Check sheet for the modelled part. Datum: model origin and axes. Units: mm. Face numbers are marked on the shaded views. A direction names the side the tool comes from. Give positions to 0.01 mm unless a question says otherwise; leave off trailing zeros. Order: outer loops, then holes, each group sorted by start corner. A loop starts at its lowest first (then second) coordinate and runs counter-clockwise, first axis right, second up. Notation, with made-up numbers: (-38, 9) -> (-7, 9) arc R12 ccw to (-7, 24) -> close; hole circle Ø11 at (59.5, -28). An arc over 180 degrees is marked (long way). Write each question's results on one line, items separated by ' | '.
from build123d import *

# Parameters (mm, degrees)
SKETCH1_R           = 16
SKETCH1_R_2         = 7.5
BOSS_EXTRUDE1_DEPTH = 4
SKETCH2_R           = 14
SKETCH2_R_2         = 9.5
CUT_EXTRUDE1_DEPTH  = 0.5
FILLET1_R           = 0.3


with BuildPart() as part:
    # Sketch1 → Boss-Extrude1 (new, symmetric)
    with BuildSketch(Plane.XY):
        Circle(SKETCH1_R)
        Circle(SKETCH1_R_2, mode=Mode.SUBTRACT)
    extrude(amount=BOSS_EXTRUDE1_DEPTH, both=True)

    # Sketch2 → Cut-Extrude1 (cut)
    with BuildSketch(Plane.XY.offset(4)):
        Circle(SKETCH2_R)
        Circle(SKETCH2_R_2, mode=Mode.SUBTRACT)
    cut_extrude1 = extrude(amount=-CUT_EXTRUDE1_DEPTH, mode=Mode.SUBTRACT)

    # Fillet1
    fillet1_edges = [part.edges().sort_by_distance(p)[0] for p in [
        (-16, 0, -4),
        (-16, 0, 4),
        (-7.5, 0, -4),
        (-7.5, 0, 4),
    ]]
    fillet(fillet1_edges, radius=FILLET1_R)

    # Mirror4: Cut-Extrude1 across plane
    add(cut_extrude1.mirror(Plane.XY), mode=Mode.SUBTRACT)


solid = part.part
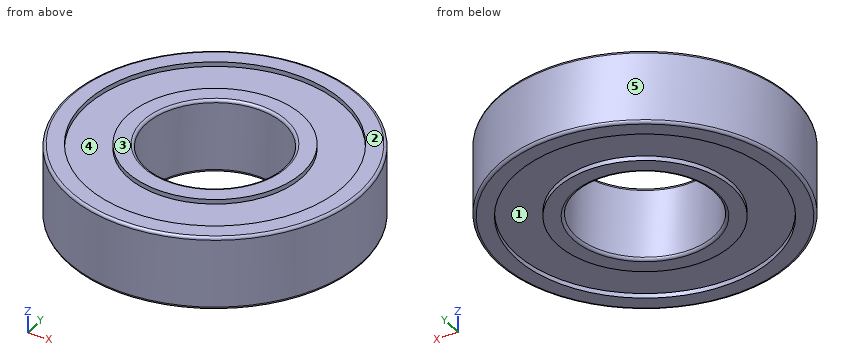
1. Access from +Z, -Z, +X, -X, +Y, -Y to the whole of each face (thin tool, end or side, straight path). Record for the marked faces 1 and 2.
Verdict:
face 1: -Z | face 2: +Z, +X, -X, +Y, -Y
2. Material ranges on probe 1 along Y at (x, z) = (0, -3.6); probe 2 along Z at (x, y) = (8.5, -7); probe 3 along X at (y, z) = (-0.5, 3.75), recorded low to high. Write a range as from..to.
Verdict:
probe 1: y = -16..-14, -9.5..-7.5, 7.5..9.5, 14..16 | probe 2: z = -3.5..3.5 | probe 3: x = -15.99..-13.99, -9.49..-7.49, 7.49..9.49, 13.99..15.99
3. Gauge pin test, flat end, axial feed: pin 1 Ø2 at (y, z) = (6.5, -1.5) entering from -X (3 decimals). Record the tip position at first contact, or that the pin passes through.
Verdict:
pin 1: stops at x = -15.025
4. Mould release check, pull along Y, two halves, no side actions. Record for the marked faces 3, 4 and 5: +Y half, -Y half, draft (parallel to the pull), parting line (faces both ways), or undercut.
Verdict:
face 3: draft | face 4: undercut | face 5: parting line
5. Section check C-C on z = -2. Record the cut outline in (x, y), then the cut area to 3 significant figures.
Verdict:
outline: circle Ø32 at (0, 0); hole circle Ø15 at (0, 0) | area: 628 mm^2
